The listing builds one solid part. Answer for the finished solid, in the listing's coordinates (mm). A direction names the side the tool comes from. Give positions to 0.01 mm unless a question says otherwise; leave off trailing zeros. Order: outer loops, then holes, each group sorted by start corner. A loop starts at its lowest first (then second) coordinate and runs counter-clockwise, first axis right, second up.
```python
from build123d import *

# Parameters (mm, degrees)
SKETCH1_R           = 8.45
BOSS_EXTRUDE1_DEPTH = 1
SKETCH4_W           = 38
SKETCH4_H           = 13.6
SKETCH4_R           = 1.8
BOSS_EXTRUDE2_DEPTH = 2


with BuildPart() as part:
    # Sketch1 → Boss-Extrude1 (new, symmetric)
    with BuildSketch(Plane.XY):
        with BuildLine():
            Line((-11.45, -12.8), (-11.45, 29.25))
            Line((-11.45, 29.25), (11.45, 29.25))
            Line((11.45, 29.25), (11.45, -12.8))
            ThreePointArc((11.45, -12.8), (0, -24.25), (-11.45, -12.8))
        make_face()
        with Locations((0, 12.8)):
            Circle(SKETCH1_R, mode=Mode.SUBTRACT)
        with Locations(Location((0, -12.8, 0), (0, 0, 180))):
            Circle(SKETCH1_R, mode=Mode.SUBTRACT)
    extrude(amount=BOSS_EXTRUDE1_DEPTH, both=True)

    # Sketch4 → Boss-Extrude2 (add)
    with BuildSketch(Plane(origin=(0, 29.25, 0), x_dir=(1, 0, 0), z_dir=(0, 1, 0))):
        with Locations((0, 5.8)):
            Rectangle(SKETCH4_W, SKETCH4_H)
        with Locations(Location((-15, 5.8, 0), (0, 0, 180))):
            Circle(SKETCH4_R, mode=Mode.SUBTRACT)
        with Locations((15, 5.8)):
            Circle(SKETCH4_R, mode=Mode.SUBTRACT)
    extrude(amount=BOSS_EXTRUDE2_DEPTH)


solid = part.part
```
1) For a pull along Z with two mould halves and no side action, classify faces 1 (the cylindrical face through (16.663, 30.236, -5.111)), 2 (the flat face through (0, 30, -12.6)), 3 (the flat face through (-19, 30, -6)) as +Z half, -Z half, draft (parallel to the pull), parting line (faces both ways), or undercut.
Geometry says:
face 1: undercut
face 2: -Z half
face 3: draft
2) Find section B-B (y = 12.8). Write down the section's boundary in (x, z).
Geometry says:
outline: (-11.45, -1) - (-8.45, -1) - (-8.45, 1) - (-11.45, 1) - close; (8.45, -1) - (11.45, -1) - (11.45, 1) - (8.45, 1) - close
3) Find section C-C (z = -5.8). Write down the section's boundary in (x, y).
Geometry says:
outline: (-19, 29.25) - (-16.8, 29.25) - (-16.8, 31.25) - (-19, 31.25) - close; (-13.2, 29.25) - (13.2, 29.25) - (13.2, 31.25) - (-13.2, 31.25) - close; (16.8, 29.25) - (19, 29.25) - (19, 31.25) - (16.8, 31.25) - close
4) Find section D-D (x = 0). Write down the section's boundary in (y, z).
Geometry says:
outline: (-24.25, -1) - (-21.25, -1) - (-21.25, 1) - (-24.25, 1) - close; (-4.35, -1) - (4.35, -1) - (4.35, 1) - (-4.35, 1) - close; (21.25, -1) - (29.25, -1) - (29.25, -12.6) - (31.25, -12.6) - (31.25, 1) - (21.25, 1) - close
5) Find section A-A (x = -15). Write down the section's boundary in (y, z).
Geometry says:
outline: (29.25, -12.6) - (31.25, -12.6) - (31.25, -7.6) - (29.25, -7.6) - close; (29.25, -4) - (31.25, -4) - (31.25, 1) - (29.25, 1) - close
6) Straight lines are drawn through the part: probe 1 along Y at (x, z) = (0, 0.6); probe 2 along Z at (x, y) = (15, 30.5); probe 3 along Z at (x, y) = (11, -11). For each, find the intervals that lie inside material, in ascending order.
Geometry says:
probe 1: y = -24.25 to -21.25, -4.35 to 4.35, 21.25 to 31.25
probe 2: z = -12.6 to -7.6, -4 to 1
probe 3: z = -1 to 1
7) A tool of negligible diameter and unlimited length cuts with its end or side. For faces 4 (the flat face through (-11.45, 8, 0)), 5 (the flat face through (11.45, 9, 0)), 6 (the flat face through (0, 3, -1)), 7 (the flat face through (0, 31.25, -6)), from which of +Z, -Z, +X, -X, +Y, -Y can it reach the whole face along a straight path? Write none if from no direction.
Geometry says:
face 4: +Z, -Z, -X, -Y
face 5: +Z, -Z, +X, -Y
face 6: -Z, +X, -X, -Y
face 7: +Z, -Z, +X, -X, +Y
8) Given P1, Ø1, axis at x = 6.5, y = -6.5, coming from the -Z side; P2, Ø3, axis at x = -15, z = -5.8, coming from the -Y side; P3, Ø1.5, axis at y = 18.5, z = -1, coming from the -X side; P4, Ø6, axis at y = -5.5, z = -1, coming from the -X side, each flat-ended and moving along its own axis, determine where each tip first touches the part or whether it passes through.
Geometry says:
P1: stops at z = -1
P2: passes through
P3: stops at x = -11.45
P4: stops at x = -11.45
